Geometry check sheet. Reference: the model listing, model coordinates, mm. A direction names the side the tool comes from. Give positions to 0.01 mm unless a question says otherwise; leave off trailing zeros. Loops run counter-clockwise (first coordinate to the right, second up) from the corner with the lowest first, then second, coordinate; pieces in that order, holes last. Notation, with made-up numbers: (57.5, -38.75) -> (74.5, -38.75) arc R21 ccw to (74.5, -8.75) -> close; hole circle Ø3 at (86.25, -15). An arc over 180 degrees is marked (long way). Answer in a Markdown table with one row per item. Add a question column.
```python
from build123d import *

# Parameters (mm, degrees)
F0_W      = 254
F0_H      = 152.4
F0_R      = 6.35
F1_DEPTH  = 25.4
F2_DEPTH  = 50.8
F3_W      = 254
F3_H      = 12.7
F4_DEPTH  = 25.4
F5_W      = 254
F5_H      = 25.4
F6_DEPTH  = 25.4
F7_W      = 254
F7_H      = 25.4
F8_DEPTH  = 25.4
F9_W      = 254
F9_H      = 25.4
F10_DEPTH = 127
F12_DEPTH = 25.4


with BuildPart() as f1:
    # F0 (on Front) → F1 (new body)
    with BuildSketch(Plane.XZ):
        Rectangle(F0_W, F0_H)
        with Locations((-50.8, 0)):
            Circle(F0_R, mode=Mode.SUBTRACT)
        with Locations((38.1, 0)):
            Circle(F0_R, mode=Mode.SUBTRACT)
    extrude(amount=F1_DEPTH)

    # F0 (on Front) → F2 (join)
    with BuildSketch(Plane.XZ):
        with Locations((38.1, 0)):
            Circle(F0_R)
        with Locations((-50.8, 0)):
            Circle(F0_R)
    extrude(amount=F2_DEPTH)

    # F3 (on face) → F4 (join, symmetric)
    with BuildSketch(Plane.XZ.offset(25.4)):
        with Locations((0, -82.55)):
            Rectangle(F3_W, F3_H)
    extrude(amount=F4_DEPTH, both=True)

    # F5 (on face) → F6 (join)
    with BuildSketch(Plane.XZ.offset(50.8)):
        with Locations((0, -76.2)):
            Rectangle(F5_W, F5_H)
    extrude(amount=F6_DEPTH)

    # F7 (on face) → F8 (cut)
    with BuildSketch(Plane.XY.offset(76.2)):
        with Locations((0, -12.7)):
            Rectangle(F7_W, F7_H)
    extrude(amount=-F8_DEPTH, mode=Mode.SUBTRACT)

    # F9 (on face) → F10 (join)
    with BuildSketch(Plane(origin=(0, 0, 0), x_dir=(-1, 0, 0), z_dir=(0, 1, 0))):
        with Locations((0, 38.1)):
            Rectangle(F9_W, F9_H)
    extrude(amount=F10_DEPTH)

    # F11 (on face) → F12 (join)
    with BuildSketch(Plane.XY.offset(50.8)):
        with BuildLine():
            ThreePointArc((44.45, 25.4), (33.6098719395, 29.8901280605), (38.1, 19.05))
            ThreePointArc((38.1, 19.05), (42.5901280605, 20.9098719395), (44.45, 25.4))
        make_face()
    extrude(amount=F12_DEPTH)


solid = f1.part
```
1. Access from +Z, -Z, +X, -X, +Y, -Y to the whole of each face (thin tool, end or side, straight path). Record for faces 1 (the face through (-2, -63, -63.5)), 2 (the face through (31.756, -37.922, 0.279)), 3 (the face through (-2, -38, -88.9)), 4 (the face through (-2, 0, -31)).
2. Sectioned sample at A-A (z = -69). Enter the section's corners in (x, y), plus the area to 3 significant figures.
3. Release check for a two-part mould opening along Z. For faces 5 (the face through (2, 63, 25.4)), 6 (the face through (-44.743, -37.922, 1.907)), 7 (the face through (38, 25, 76.2)), 8 (the face through (-127, -5, -4)) record: released by +Z, released by -Z, zero draft, split by the parting line, or undercut.
4. Sectioned sample at D-D (z = 0). Enter the section's corners in (x, y).
5. Gauge pin test, flat ends, axial feed: pin 1 Ø14 at (x, z) = (-8.5, -67) entering from +Y; pin 2 Ø1.5 at (x, z) = (-77.5, 0) entering from -Y; pin 3 Ø1 at (x, y) = (-58.5, 105) entering from -Z. Record the tip position at first contact, or that the pin passes through.
6. Material ranges on L1, parallel to Y at x = -23.5, z = -74.5; L2, parallel to Z at x = -109.5, y = 40; L3, parallel to Y at x = 13.5, z = 18, recorded low to high. Write a range as from..to.
7. Sectioned sample at B-B (y = -42). Enter the section's corners in (x, z), plus the area to 3 significant figures.
8. Sectioned sample at C-C (x = -13). Enter the section's corners in (y, z).
Response:
| question | item | result |
|---|---|---|
| 1 | face 1 | +Z, +X, -X, -Y |
| 1 | face 2 | -Y |
| 1 | face 3 | -Z, +X, -X, +Y, -Y |
| 1 | face 4 | -Z, +X, -X, +Y |
| 2 | outline | (-127, -76.2) -> (127, -76.2) -> (127, -50.8) -> (-127, -50.8) -> close; (-127, -25.4) -> (127, -25.4) -> (127, 0) -> (-127, 0) -> close |
| 2 | area | 12,900 mm2 |
| 3 | face 5 | released by -Z |
| 3 | face 6 | undercut |
| 3 | face 7 | released by +Z |
| 3 | face 8 | zero draft |
| 4 | outline | (-127, -25.4) -> (-57.15, -25.4) -> (-57.15, -50.8) -> (-44.45, -50.8) -> (-44.45, -25.4) -> (31.75, -25.4) -> (31.75, -50.8) -> (44.45, -50.8) -> (44.45, -25.4) -> (127, -25.4) -> (127, 0) -> (-127, 0) -> close |
| 5 | pin 1 | stops at y = 0 |
| 5 | pin 2 | stops at y = -25.4 |
| 5 | pin 3 | stops at z = 25.4 |
| 6 | L1 | y = -76.2..-50.8, -25.4..0 |
| 6 | L2 | z = 25.4..50.8 |
| 6 | L3 | y = -25.4..0 |
| 7 | outline | (-127, -88.9) -> (127, -88.9) -> (127, -76.2) -> (-127, -76.2) -> close; circle Ø12.7 at (-50.8, 0); circle Ø12.7 at (38.1, 0) |
| 7 | area | 3,480 mm2 |
| 8 | outline | (-76.2, -88.9) -> (0, -88.9) -> (0, 25.4) -> (127, 25.4) -> (127, 50.8) -> (-25.4, 50.8) -> (-25.4, -76.2) -> (-50.8, -76.2) -> (-50.8, -63.5) -> (-76.2, -63.5) -> close |
